The figure shows three views and two pictorial views of one solid part (mm, origin at its lowest corner). Answer the questions. Give positions to 0.01 mm unless a question says otherwise; leave off trailing zeros. Loops run counter-clockwise (first coordinate to the right, second up) from the corner with the lowest first, then second, coordinate; pieces in that order, holes last. Notation, with made-up numbers: (1, -29) - (60, -29) arc R23 ccw to (60, -5) - close; hole circle Ø5 at (47, 77.5). An arc over 180 degrees is marked (long way). One line per question, with ' | ' between items.
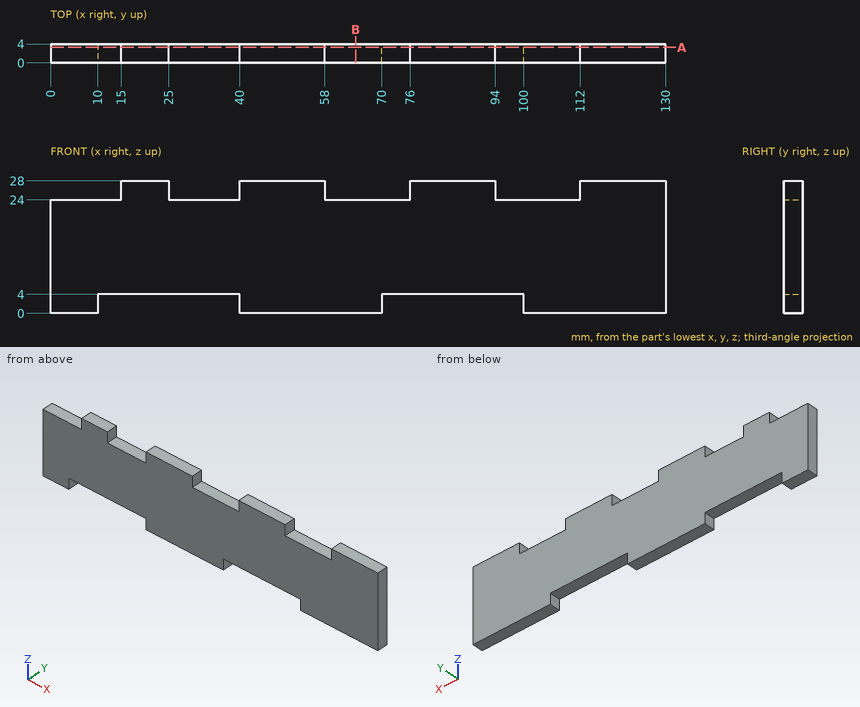
1. Consider L1, parallel to X at y = 3.7, z = 26.25; L2, parallel to X at y = 2.4, z = 1.5; L3, parallel to Z at x = 94.5, y = 3.7. Determine where each line is inside the solid, lowest interval first.
Evaluation:
L1: 15 to 25, 40 to 58, 76 to 94, 112 to 130 | L2: 0 to 10, 40 to 70, 100 to 130 | L3: 4 to 24
2. Find section A-A on y = 3.3. Write down the section's boundary in (x, z), then the cut area to 3 significant figures.
Evaluation:
outline: (0, 0) - (10, 0) - (10, 4) - (40, 4) - (40, 0) - (70, 0) - (70, 4) - (100, 4) - (100, 0) - (130, 0) - (130, 28) - (112, 28) - (112, 24) - (94, 24) - (94, 28) - (76, 28) - (76, 24) - (58, 24) - (58, 28) - (40, 28) - (40, 24) - (25, 24) - (25, 28) - (15, 28) - (15, 24) - (0, 24) - close | area: 3,140 mm2
3. Flat-ended cylindrical pins translate along their axes: pin 1 (2 mm diameter, centred on y = 3, z = 25.5, fed in from -X); pin 2 (1.2 mm diameter, centred on x = 64, y = 2.5, fed in from +Z); pin 3 (1.2 mm diameter, centred on x = 28.5, y = 1.5, fed in from -Z). Find the tip coordinate at first contact, or state that the pin passes through.
Evaluation:
pin 1: x = 15 | pin 2: z = 24 | pin 3: z = 4
4. Find section B-B on x = 64.5. Write down the section's boundary in (y, z), then the cut area to 3 significant figures.
Evaluation:
outline: (0, 0) - (4, 0) - (4, 24) - (0, 24) - close | area: 96.0 mm2
